Source: CAD feature listing. Evaluate the final solid. Frame: model axes, mm. A direction names the side the tool comes from. Round coordinates to 2 decimals unless told otherwise and drop trailing zeros. Write each loop counter-clockwise with the first axis right and the second up, starting at its lowest first coordinate (ties: lowest second). Pieces come first, ordered by that corner, then holes. Notation, with made-up numbers: M 31.25,4.25 L 81.25,4.25 A24 ccw 81.25,28.25 Z; hole C 53,88.5 d10. An arc over 180 degrees is marked long. Put each result on its own line as item: value. Start each with the question number.
Autodesk Inventor part; units mm, degrees
ref_plane "YZ Plane" through (0, 0, 0) normal (1, 0, 0) x (0, 1, 0)
ref_plane "XZ Plane" through (0, 0, 0) normal (0, 1, 0) x (-1, 0, 0)
ref_plane "XY Plane" through (0, 0, 0) normal (0, 0, 1) x (1, 0, 0)
sketch "Sketch1" plane through (0, 0, 0) normal (0, 0, 1) x (1, 0, 0)
  line L0 (85.72, 30.226) -> (85.72, 1.401) construction
  line L1 (85.72, 1.401) -> (45.72, 1.401) construction
  line L2 (85.72, 1.401) -> (5.72, 1.401) construction
  line L3 (5.72, 1.401) -> (5.72, 59.001) construction
  line L4 (5.72, 59.001) -> (85.72, 59.001) construction
  line L5 (85.72, 59.001) -> (85.72, 1.401) construction
  line L6 (61.99, 1.401) -> (61.99, 20.221) construction
  line L7 (61.99, 20.221) -> (85.72, 20.221) construction
  line L8 (61.99, 20.221) -> (58.44, 20.221) construction
  line L9 (61.99, 23.771) -> (61.99, 20.221) construction
  line L10 (60.215, 20.221) -> (61.99, 20.221) construction
  line L11 (61.99, 20.221) -> (61.99, 21.996) construction
  line L12 (61.99, 21.996) -> (60.215, 21.996) construction
  line L13 (60.215, 21.996) -> (60.215, 20.221) construction
  circle A0 centre (60.215, 21.996) radius 1.775 construction
  circle A1 centre (60.215, 21.996) radius 2.775 construction
  circle A2 centre (60.215, 21.996) radius 4.275 construction
  line L14 (5.72, 59.001) -> (74.72, 59.001) construction
  line L15 (74.72, 59.001) -> (74.72, 53.301) construction
  line L16 (74.72, 53.301) -> (5.72, 53.301) construction
  line L17 (5.72, 53.301) -> (5.72, 59.001) construction
  line L18 (5.72, 1.401) -> (18.72, 1.401) construction
  line L19 (18.72, 1.401) -> (18.72, 14.401) construction
  line L20 (18.72, 14.401) -> (5.72, 14.401) construction
  line L21 (5.72, 14.401) -> (5.72, 1.401) construction
  circle A3 centre (2.72, 58.001) radius 1.5
  line L22 (3.72, 61.001) -> (5.72, 61.001)
  line L23 (5.72, 61.001) -> (5.72, 59.001) construction
  line L24 (5.72, 61.001) -> (2.72, 61.001)
  line L25 (5.72, 55.001) -> (5.72, 61.001) construction
  line L26 (45.72, 1.9437) -> (45.72, 30.226) construction
  line L27 (45.72, 30.226) -> (85.72, 30.226) construction
  arc A4 (2.72, 61.001) -> (1.52, 55.2515) centre (2.72, 58.001) ccw
  circle A5 centre (2.72, 2.451) radius 1.5
  line L28 (3.72, -0.549) -> (5.72, -0.549)
  line L29 (5.72, -0.549) -> (2.72, -0.549)
  arc A6 (1.52, 5.2005) -> (2.72, -0.549) centre (2.72, 2.451) ccw
  circle A7 centre (88.72, 58.001) radius 1.5
  line L30 (85.72, 61.001) -> (88.72, 61.001)
  arc A8 (89.92, 55.2515) -> (88.72, 61.001) centre (88.72, 58.001) ccw
  line L31 (85.72, -0.549) -> (88.72, -0.549)
  circle A9 centre (88.72, 2.451) radius 1.5
  arc A10 (88.72, -0.549) -> (89.92, 5.2005) centre (88.72, 2.451) ccw
  line L32 (2.72, 53.4184) -> (2.72, 7.0336)
  line L33 (5.72, 61.001) -> (85.72, 61.001)
  line L34 (88.72, 53.4184) -> (88.72, 7.0336)
  line L35 (85.72, -0.549) -> (5.72, -0.549)
  arc A11 (2.72, 53.4184) -> (1.52, 55.2515) centre (0.72, 53.4184) ccw
  arc A12 (1.52, 5.2005) -> (2.72, 7.0336) centre (0.72, 7.0336) ccw
  arc A13 (88.72, 7.0336) -> (89.92, 5.2005) centre (90.72, 7.0336) ccw
  arc A14 (89.92, 55.2515) -> (88.72, 53.4184) centre (90.72, 53.4184) ccw
  point P0 (0, 0)
  point P1 (2.72, 55.001)
  point P2 (2.72, 5.451)
  point P3 (91.44, 0)
  point P4 (88.72, 55.001)
  point P5 (88.72, 5.451)
  dimension "d32" = 40
  dimension "d33" = 28.825
  dimension "d34" = 80
  dimension "d37" = 18.82
  dimension "d40" = 5.55
  dimension "d41" = 8.55
  dimension "d42" = 69
  dimension "d43" = 5.7
  dimension "d44" = 13
  dimension "d45" = 13
  dimension "d52" = 2
  dimension "d80" = 3
extrude "Extrusion1" add sketch "Sketch1" along normal blind 2
sketch "Sketch2" plane through (0, 0, 2) normal (0, 0, 1) x (1, 0, 0)
  line L0 (85.72, 30.226) -> (85.72, 1.401)
  line L1 (5.72, 14.401) -> (5.72, 53.301)
  line L2 (74.72, 59.001) -> (85.72, 59.001)
  line L3 (85.72, 59.001) -> (85.72, 1.401)
  line L4 (61.815, 21.996) -> (60.215, 21.996)
  circle A0 centre (60.215, 21.996) radius 1.6
  circle A1 centre (60.215, 21.996) radius 2.775 construction
  circle A2 centre (60.215, 21.996) radius 4.275
  line L5 (45.72, 59.001) -> (74.72, 59.001)
  line L6 (74.72, 59.001) -> (74.72, 53.301)
  line L7 (74.72, 53.301) -> (5.72, 53.301)
  line L8 (5.72, 58.001) -> (5.72, 59.001)
  line L9 (5.72, 1.401) -> (18.72, 1.401)
  line L10 (18.72, 1.401) -> (18.72, 14.401)
  line L11 (18.72, 14.401) -> (5.72, 14.401)
  line L12 (5.72, 2.451) -> (5.72, 1.401)
  circle A3 centre (2.72, 58.001) radius 1.5
  line L13 (3.72, 61.001) -> (5.72, 61.001)
  line L14 (5.72, 61.001) -> (5.72, 59.001)
  line L15 (5.72, 61.001) -> (2.72, 61.001)
  line L16 (5.72, 59.001) -> (5.72, 61.001)
  arc A4 (2.72, 61.001) -> (1.52, 55.2515) centre (2.72, 58.001) ccw
  line L17 (3.72, -0.549) -> (5.72, -0.549)
  line L18 (5.72, -0.549) -> (2.72, -0.549)
  circle A5 centre (2.72, 2.451) radius 1.5
  arc A6 (1.52, 5.2005) -> (2.72, -0.549) centre (2.72, 2.451) ccw
  line L19 (85.72, -0.549) -> (88.72, -0.549)
  circle A7 centre (88.72, 2.451) radius 1.5
  arc A8 (88.72, -0.549) -> (89.92, 5.2005) centre (88.72, 2.451) ccw
  circle A9 centre (88.72, 58.001) radius 1.5
  arc A10 (89.92, 55.2515) -> (88.72, 61.001) centre (88.72, 58.001) ccw
  line L20 (85.72, 61.001) -> (88.72, 61.001)
  line L21 (2.72, 53.4184) -> (2.72, 7.0336)
  line L22 (5.72, 61.001) -> (85.72, 61.001)
  line L23 (88.72, 53.4184) -> (88.72, 7.0336)
  line L24 (85.72, -0.549) -> (5.72, -0.549)
  arc A11 (2.72, 53.4184) -> (1.52, 55.2515) centre (0.72, 53.4184) ccw
  arc A12 (1.52, 5.2005) -> (2.72, 7.0336) centre (0.72, 7.0336) ccw
  arc A13 (88.72, 7.0336) -> (89.92, 5.2005) centre (90.72, 7.0336) ccw
  arc A14 (89.92, 55.2515) -> (88.72, 53.4184) centre (90.72, 53.4184) ccw
  line L25 (85.72, 1.401) -> (74.72, 1.401)
  line L26 (61.99, 1.401) -> (45.72, 1.401)
  line L27 (85.72, 1.401) -> (74.72, 1.401)
  line L28 (61.99, 1.401) -> (18.72, 1.401)
  line L29 (61.99, 1.401) -> (74.72, 1.401)
  point P0 (0, 0)
  point P1 (2.72, 55.001)
  point P2 (2.72, 5.451)
  point P3 (91.44, 0)
  point P4 (88.72, 5.451)
  point P5 (88.72, 55.001)
  dimension "d89" = 3.2
  dimension "d53" = 40
  dimension "d54" = 28.825
  dimension "d55" = 80
  dimension "d57" = 5.55
  dimension "d58" = 8.55
  dimension "d59" = 69
  dimension "d60" = 5.7
  dimension "d61" = 13
  dimension "d62" = 13
  dimension "d63" = 2
  dimension "d81" = 3
  dimension "d82" = 3
  dimension "d83" = 3
  dimension "d84" = 3
extrude "Extrusion2" add sketch "Sketch2" along normal blind 3
sketch "Sketch5" plane through (0, 0, 5) normal (0, 0, 1) x (1, 0, 0)
  line L0 (85.72, 30.226) -> (85.72, 1.401)
  line L1 (85.72, 1.401) -> (45.72, 1.401)
  line L2 (85.72, 1.401) -> (5.72, 1.401)
  line L3 (5.72, 1.401) -> (5.72, 59.001)
  line L4 (5.72, 59.001) -> (85.72, 59.001)
  line L5 (85.72, 59.001) -> (85.72, 1.401)
  line L6 (5.72, 59.001) -> (74.72, 59.001)
  line L7 (5.72, 53.301) -> (5.72, 59.001)
  line L8 (5.72, 1.401) -> (18.72, 1.401)
  line L9 (5.72, 14.401) -> (5.72, 1.401)
  circle A0 centre (2.72, 58.001) radius 1.5
  line L10 (3.72, 61.001) -> (5.72, 61.001)
  line L11 (5.72, 61.001) -> (5.72, 59.001)
  line L12 (5.72, 61.001) -> (2.72, 61.001)
  line L13 (5.72, 55.001) -> (5.72, 61.001)
  arc A1 (2.72, 61.001) -> (1.52, 55.2515) centre (2.72, 58.001) ccw
  line L14 (3.72, -0.549) -> (5.72, -0.549)
  line L15 (5.72, -0.549) -> (2.72, -0.549)
  circle A2 centre (2.72, 2.451) radius 1.5
  arc A3 (1.52, 5.2005) -> (2.72, -0.549) centre (2.72, 2.451) ccw
  line L16 (85.72, -0.549) -> (88.72, -0.549)
  circle A4 centre (88.72, 2.451) radius 1.5
  arc A5 (88.72, -0.549) -> (89.92, 5.2005) centre (88.72, 2.451) ccw
  circle A6 centre (88.72, 58.001) radius 1.5
  arc A7 (89.92, 55.2515) -> (88.72, 61.001) centre (88.72, 58.001) ccw
  line L17 (85.72, 61.001) -> (88.72, 61.001)
  line L18 (2.72, 53.4184) -> (2.72, 7.0336)
  line L19 (5.72, 61.001) -> (85.72, 61.001)
  line L20 (88.72, 53.4184) -> (88.72, 7.0336)
  line L21 (85.72, -0.549) -> (5.72, -0.549)
  arc A8 (2.72, 53.4184) -> (1.52, 55.2515) centre (0.72, 53.4184) ccw
  arc A9 (1.52, 5.2005) -> (2.72, 7.0336) centre (0.72, 7.0336) ccw
  arc A10 (88.72, 7.0336) -> (89.92, 5.2005) centre (90.72, 7.0336) ccw
  arc A11 (89.92, 55.2515) -> (88.72, 53.4184) centre (90.72, 53.4184) ccw
  point P0 (0, 0)
  point P1 (0, 0)
  point P2 (2.72, 55.001)
  point P3 (2.72, 5.451)
  point P4 (91.44, 0)
  point P5 (88.72, 5.451)
  point P6 (88.72, 55.001)
  dimension "d64" = 40
  dimension "d65" = 28.825
  dimension "d66" = 80
  dimension "d74" = 2
  dimension "d85" = 3
  dimension "d86" = 3
  dimension "d87" = 3
  dimension "d88" = 3
extrude "Extrusion5" add sketch "Sketch5" along normal blind 1.67
chamfer "Chamfer1" distance 1 distance2 3 1 edges at (55.94, 21.996, 5) measured on face at (63.5414, 21.5273, 5)
sketch "Sketch6" plane through (2.72, -0.549, 0) normal (0, -1, 0) x (1, 0, 0)
  line L0 (-2.72, 20.7114) -> (-2.72, 7.1986) construction
  arc A0 (14.6348, 17.447) -> (18.9452, 17.447) centre (16.79, 14.78) ccw construction
  line L1 (14.6347, 17.447) -> (18.9453, 17.447) construction
  line L2 (-3, 20.67) -> (-3, 6.67) construction
  line L3 (0, 13.555) -> (92, 13.555) construction
  line L4 (0.28, 13.555) -> (46, 13.555) construction
  line L5 (13.7208, 18.67) -> (19.8592, 18.67)
  line L6 (8.6741, 18.67) -> (83, 18.67) construction
  line L7 (83, 18.67) -> (8.6741, 18.67) construction
  circle A1 centre (16.79, 14.78) radius 7.15 construction
  circle A2 centre (16.79, 14.78) radius 6.25 construction
  line L8 (18.077, 2.0446) -> (21.077, 2.0446)
  line L9 (13.0545, 18.0609) -> (13.0545, 18.67) construction
  line L10 (11.835, 14.78) -> (11.4131, 5.117) construction
  line L11 (11.835, 14.78) -> (21.5072, 14.78) construction
  line L12 (21.745, 14.78) -> (22.1562, 5.3611) construction
  line L13 (21.745, 14.78) -> (31.1729, 14.78) construction
  arc A3 (13.7208, 18.67) -> (21.5912, 13.555) centre (16.79, 14.78) ccw
  arc A4 (21.5912, 13.555) -> (19.8592, 18.67) centre (16.79, 14.78) ccw
  line L14 (22.1562, 5.3611) -> (11.4131, 5.117) construction
  line L15 (-3, 20.67) -> (-3, 6.67)
  line L16 (0, 6.67) -> (-3, 6.67)
  arc A5 (9.985, 20.67) -> (23.595, 20.67) centre (16.79, 14.78) ccw
  line L17 (16.79, 14.78) -> (7.79, 14.78) construction
  line L18 (7.79, 14.78) -> (7.79, 0)
  line L19 (86, 0) -> (0, 0)
  line L20 (16.79, 14.78) -> (25.79, 14.78) construction
  line L21 (25.79, 14.78) -> (25.79, 0)
  line L22 (-3, 20.67) -> (-2.72, 20.67)
  line L23 (9.985, 20.67) -> (35.5259, 20.67)
  point P0 (-2.72, 0)
  point P1 (-2.72, 20.67)
  point P2 (-1.2, 6.67)
  dimension "d90" = 14.3
  dimension "d91" = 12.5
  dimension "d92" = 3
  dimension "d93" = 92.5
  dimension "d94" = 87.5
extrude "Extrusion6" add sketch "Sketch6" along normal blind 8
sketch "Sketch7" plane through (2.72, -8.549, 0) normal (0, -1, 0) x (1, 0, 0)
  point P0 (-2.72, 0)
sketch "Sketch8" plane through (2.72, -0.549, 0) normal (0, 1, 0) x (1, 0, 0)
  line L0 (18.077, 2.0446) -> (21.077, 2.0446)
  line L1 (86, 0) -> (0, 0) construction
  line L2 (22.1562, -5.3611) -> (11.4131, -5.117) construction
  line L3 (18.077, -2.0446) -> (21.077, -2.0446) construction
  line L4 (-2.72, -20.7114) -> (-2.72, -7.1986) construction
  line L5 (-3, -20.67) -> (-3, -6.67) construction
  line L6 (-3, -20.67) -> (-3, -6.67)
  line L7 (0, -13.555) -> (92, -13.555) construction
  line L8 (0.28, -13.555) -> (46, -13.555) construction
  line L9 (0, -6.67) -> (-3, -6.67)
  line L10 (7.79, -14.78) -> (7.79, 0) construction
  line L11 (25.79, -14.78) -> (25.79, 0) construction
  line L12 (-3, -20.67) -> (-2.72, -20.67)
  line L13 (13.04, -8.2848) -> (20.54, -8.2848) construction
  line L14 (20.54, -8.2848) -> (24.29, -14.78) construction
  line L15 (22.415, -11.5324) -> (28.3907, -11.5324) construction
  line L16 (27.6858, -27.8063) -> (6.6122, -26.5118)
  line L17 (6.6122, -26.5118) -> (5.8176, -11.5324)
  arc A0 (21.5912, -13.555) -> (20.5323, -11.5324) centre (16.79, -14.78) ccw construction
  line L18 (28.3907, -11.5324) -> (23.5504, -11.5324)
  line L19 (10.0296, -11.5324) -> (5.8176, -11.5324)
  arc A1 (23.5504, -11.5324) -> (10.0296, -11.5324) centre (16.79, -14.78) ccw
  line L20 (28.3907, -11.5324) -> (27.6858, -27.8063)
  point P0 (-2.72, 0)
  point P1 (-2.72, 0)
  point P2 (-2.72, -20.67)
  point P3 (-1.2, -6.67)
extrude "Extrusion7" cut sketch "Sketch8" against normal blind 5
properties part number "Redid DAQ Enclosure Bottom TTL"
(1) Section query A-A (y = 15.5). Return loops of the section in (x, z).
(2) Section query C-C (z = 17.25). Return loops of the section in (x, y).
(3) Contact query for flat-ended pins moving along their axis: P1, Ø6, axis at x = 60.5, y = 16, coming from the +Z side; P2, Ø1.4, axis at y = 44, z = 4.5, coming from the -X side; P3, Ø3, axis at x = 32.5, y = 34.5, coming from the +Z side; P4, Ø6, axis at y = 3, z = 6.5, coming from the +X side. Output: stop coordinate, or through.
(4) Section query B-B (x = 53). Return loops of the section in (y, z), and give its area (3 significant figures).
(5) Section query D-D (x = 76.5). Return loops of the section in (y, z), and give its area (3 significant figures).
(6) Pull-direction query (Y, two-part tool) for faces 6 (the flat face through (5.72, 30, 4)), 7 (the cylindrical face through (24.19, -7.03, 16.41)), 8 (the flat face through (46, 1.401, 4)), 9 (the flat face through (19, -0.549, 7)); classes: +Y half, -Y half, draft (parallel to the pull), parting line (faces both ways), or undercut.
(7) Access query for faces 1 (the flat face through (19, -7, 18.67)), 2 (the cylindrical face through (2.4, 54.5, 3.3)), 3 (the flat face through (28.51, -4, 6)), 4 (the cylindrical face through (89.04, 54.5, 3.29)), 5 (the flat face through (41, 53.301, 3)). Directions: +Z, -Z, +X, -X, +Y, -Y. A direction counts if a zero-diameter tool reaches every point of the face in a straight line with its end or side. Return the directions, or none.
(8) Ray query, line 1 along Y through (x, z) = (21, 6.25); line 2 along X through (y, z) = (31.5, 5.25); line 3 along Z through (x, y) = (47, 5.5). Return the intervals inside material, ascending.
Entries:
1. outline: M 2.72,0 L 88.72,0 L 88.72,6.67 L 85.72,6.67 L 85.72,2 L 5.72,2 L 5.72,6.67 L 2.72,6.67 Z
2. outline: M 10.86,-8.55 L 15.21,-8.55 L 15.21,-5.55 L 10.86,-5.55 Z; M 23.81,-8.55 L 28.16,-8.55 L 28.16,-5.55 L 23.81,-5.55 Z
3. P1: z = 5
3. P2: x = 2.72
3. P3: z = 2
3. P4: x = 91.72
4. outline: M -0.55,0 L 61,0 L 61,6.67 L 59,6.67 L 59,5 L 53.3,5 L 53.3,2 L 1.4,2 L 1.4,6.67 L -0.55,6.67 Z
4. area: 159 mm2
5. outline: M -0.55,0 L 61,0 L 61,6.67 L 59,6.67 L 59,2 L 1.4,2 L 1.4,6.67 L -0.55,6.67 Z
5. area: 142 mm2
6. face 6: undercut
6. face 7: draft
6. face 8: undercut
6. face 9: +Y half
7. face 1: +Y, -Y
7. face 2: +Z, -Z, -X
7. face 3: +Z, -Z, +X, -Y
7. face 4: +Z, -Z, +X
7. face 5: +Z
8. line 1: -8.55 to 1.4, 59 to 61
8. line 2: 2.72 to 5.72, 85.72 to 88.72
8. line 3: 0 to 2
